The listing builds one solid part. Answer for the finished solid, in the listing's coordinates (mm). Face numbers are marked on the shaded views. A direction names the side the tool comes from. Coordinates: 2 decimals unless noted, no trailing zeros. Write each loop counter-clockwise with the first axis right and the second up, starting at its lowest first coordinate (ties: lowest second). Pieces come first, ordered by that corner, then holes.
(1) The part is cut by section B-B on x = 0. Give the number of separate pieces and of enclosed holes in the cut face, plus the area to 3 significant figures.
(2) The part is cut by section D-D on z = 3.5. Determine the outline of the cut face in (x, y) (3 decimals).
(3) Which of the six approach directions +Z, -Z, +X, -X, +Y, -Y give full straight-line access (tool end or side, diameter ignored) to the marked faces 4, 5 and 6?
(4) Straight lines are drawn through the part: line 1 (Y direction, x = 0, z = 3.5) (3 decimals); line 2 (Y direction, x = 0, z = 6.5) (3 decimals); line 3 (X direction, y = -4.5, z = 0.25). For each, find the intervals that lie inside material, in ascending order.
(5) The part is cut by section C-C on y = 5.75. Determine the outline of the cut face in (x, z), plus the area to 3 significant figures.
(6) The part is cut by section A-A on z = 8.5. Determine the outline of the cut face in (x, y) (3 decimals).
(7) Given P1, Ø5, axis at x = 9.96, y = 5.75, coming from the +Z side; P2, Ø1.5, axis at x = -10.5, y = -10.5, coming from the -Z side; P3, Ø3, axis at x = 9.96, y = -5.75, coming from the -Z side; P4, Ø4, axis at x = -11, z = 9, coming from the +Y side, each flat-ended and moving along its own axis, determine where each tip first touches the part or whether it passes through.
(8) For a pull along Y with two mould halves and no side action, classify the marked faces 1, 2 and 3 as +Y half, -Y half, draft (parallel to the pull), parting line (faces both ways), or undercut.
from build123d import *

# Parameters (mm, degrees)
SKETCH2_R           = 15.5
SKETCH2_R_2         = 1.625
BOSS_EXTRUDE1_DEPTH = 10
SKETCH3_R           = 7.425
BOSS_EXTRUDE2_DEPTH = 5.5
BOSS_EXTRUDE4_START = 5.5
SKETCH6_R           = 7.425
BOSS_EXTRUDE4_DEPTH = 5.5
SKETCH7_R           = 2
BOSS_EXTRUDE5_DEPTH = 1
FILLET2_R           = 0.05
CUT_EXTRUDE1_DEPTH  = 11


with BuildPart() as part:
    # Sketch2 → Boss-Extrude1 (new body)
    with BuildSketch(Plane.XY):
        Circle(SKETCH2_R)
        with Locations((0, 11.5)):
            Circle(SKETCH2_R_2, mode=Mode.SUBTRACT)
        with Locations((9.959292144, 5.75)):
            Circle(SKETCH2_R_2, mode=Mode.SUBTRACT)
        with Locations((9.959292144, -5.75)):
            Circle(SKETCH2_R_2, mode=Mode.SUBTRACT)
        with Locations((0, -11.5)):
            Circle(SKETCH2_R_2, mode=Mode.SUBTRACT)
        with Locations((-9.959292144, -5.75)):
            Circle(SKETCH2_R_2, mode=Mode.SUBTRACT)
        with Locations((-9.959292144, 5.75)):
            Circle(SKETCH2_R_2, mode=Mode.SUBTRACT)
    extrude(amount=BOSS_EXTRUDE1_DEPTH)

    # Sketch3 → Boss-Extrude2 (add)
    with BuildSketch(Plane.XY.offset(10)):
        Circle(SKETCH3_R)
    extrude(amount=BOSS_EXTRUDE2_DEPTH)

    # Sketch6 → Boss-Extrude4 (add)
    with BuildSketch(Plane(origin=(0, 0, 0), x_dir=(-1, 0, 0), z_dir=(0, 0, -1)).offset(BOSS_EXTRUDE4_START)):
        with Locations(Location((0, 0, 0), (0, 0, 180))):
            Circle(SKETCH6_R)
    extrude(amount=-BOSS_EXTRUDE4_DEPTH)

    # Sketch7 → Boss-Extrude5 (add)
    with BuildSketch(Plane(origin=(0, 0, -5.5), x_dir=(-1, 0, 0), z_dir=(0, 0, -1))):
        Circle(SKETCH7_R)
    extrude(amount=BOSS_EXTRUDE5_DEPTH)

    # Fillet2
    fillet2_edges = [part.edges().sort_by_distance(p)[0] for p in [
        (2, 0, -6.5),
    ]]
    fillet(fillet2_edges, radius=FILLET2_R)

    # Sketch9 → Cut-Extrude1 (cut)
    with BuildSketch(Plane(origin=(0, 0, -6.5), x_dir=(-1, 0, 0), z_dir=(0, 0, -1))):
        with BuildLine():
            Line((-1.224744871, 1.25), (1.224744871, 1.25))
            ThreePointArc((1.224744871, 1.25), (0, -1.75), (-1.224744871, 1.25))
        make_face()
    extrude(amount=-CUT_EXTRUDE1_DEPTH, mode=Mode.SUBTRACT)


solid = part.part
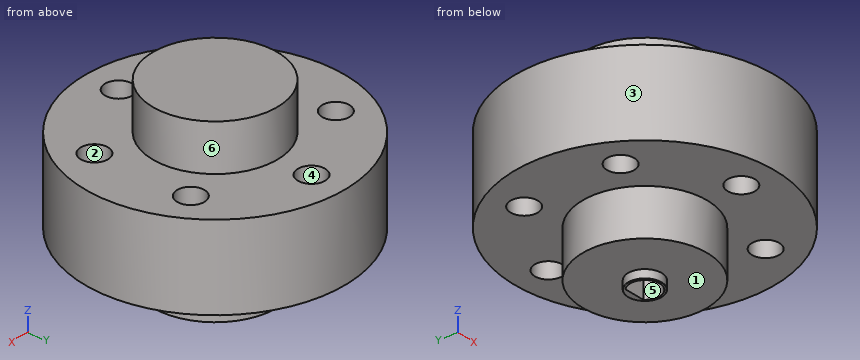
Model answer:
1. separate pieces: 3
1. enclosed holes: 0
1. area: 379 mm2
2. outline: circle Ø31 at (0, 0); hole circle Ø3.25 at (-9.959, -5.75); hole circle Ø3.25 at (-9.959, 5.75); hole circle Ø3.25 at (0, -11.5); hole circle Ø3.25 at (0, 11.5); hole (-1.225, 1.25) arc R1.75 ccw (long way) to (1.225, 1.25) - close; hole circle Ø3.25 at (9.959, -5.75); hole circle Ø3.25 at (9.959, 5.75)
3. face 4: +Z, -Z
3. face 5: -Z
3. face 6: +Z
4. line 1: y = -15.5 to -13.125, -9.875 to -1.75, 1.25 to 9.875, 13.125 to 15.5
4. line 2: y = -15.5 to -13.125, -9.875 to 9.875, 13.125 to 15.5
4. line 3: x = -14.83 to -11, -8.92 to 8.92, 11 to 14.83
5. outline: (-14.39, 0) - (-11.58, 0) - (-11.58, 10) - (-14.39, 10) - close; (-8.33, 0) - (-4.7, 0) - (-4.7, -5.5) - (4.7, -5.5) - (4.7, 0) - (8.33, 0) - (8.33, 10) - (4.7, 10) - (4.7, 15.5) - (-4.7, 15.5) - (-4.7, 10) - (-8.33, 10) - close; (11.58, 0) - (14.39, 0) - (14.39, 10) - (11.58, 10) - close
5. area: 326 mm2
6. outline: circle Ø31 at (0, 0); hole circle Ø3.25 at (-9.959, -5.75); hole circle Ø3.25 at (-9.959, 5.75); hole circle Ø3.25 at (0, -11.5); hole circle Ø3.25 at (0, 11.5); hole circle Ø3.25 at (9.959, -5.75); hole circle Ø3.25 at (9.959, 5.75)
7. P1: stops at z = 10
7. P2: stops at z = 0
7. P3: passes through
7. P4: stops at y = 12.62
8. face 1: draft
8. face 2: undercut
8. face 3: parting line
